Geometry check sheet. Reference: the model listing, model coordinates, mm. Round coordinates to 2 decimals unless told otherwise and drop trailing zeros. Loops run counter-clockwise (first coordinate to the right, second up) from the corner with the lowest first, then second, coordinate; pieces in that order, holes last. Notation, with made-up numbers: (85, 2) -> (141, 2) arc R10 cw to (141, 21) -> close; hole circle Ø10 at (36.5, -18.75). An arc over 180 degrees is marked (long way). Use a Markdown table: item, result. Add a question column.
Q1. Gauge pin test, flat ends, axial feed: P1, Ø2.5, axis at x = -25, z = 1.5, coming from the +Y side; P2, Ø3, axis at x = 4.5, z = 3, coming from the +Y side; P3, Ø2.5, axis at y = -17.5, z = 1.5, coming from the +X side. Record the tip position at first contact, or that the pin passes through.
Q2. Sectioned sample at D-D, the plane y = 51.5. Enter the section's corners in (x, z), then the cut area to 3 significant figures.
Q3. Material ranges on L1, parallel to Y at x = 0, z = 2.6; L2, parallel to Y at x = 11, z = 1.4; L3, parallel to X at y = 11.5, z = 2.3, recorded low to high.
Q4. Sectioned sample at A-A, the plane y = 0. Enter the section's corners in (x, z), then the cut area to 3 significant figures.
Q5. Sectioned sample at C-C, the plane z = 3.65. Enter the section's corners in (x, y), then the cut area to 3 significant figures.
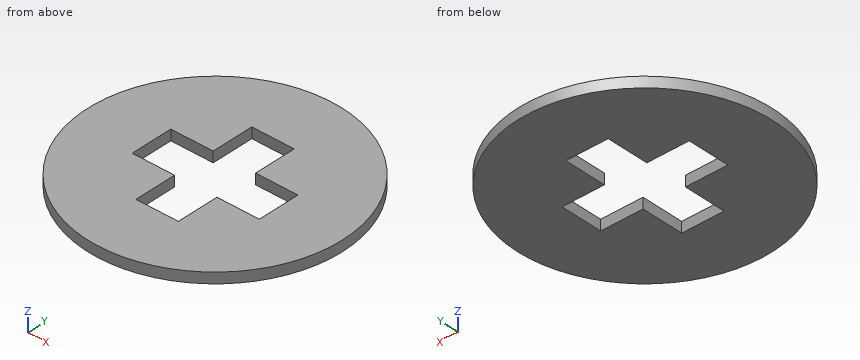
```python
from build123d import *

# Parameters (mm, degrees)
F0_R     = 60
F1_DEPTH = 5


with BuildPart() as f1:
    # F0 (on Top) → F1 (new body)
    with BuildSketch(Plane.XY):
        Circle(F0_R)
        Polygon((-10, 30), (0, 30), (10, 30), (10, 10), (30, 10), (30, 0), (30, -10), (10, -10), (10, -30), (0, -30), (-10, -30), (-10, -10), (-30, -10), (-30, 0), (-30, 10), (-10, 10), align=None, mode=Mode.SUBTRACT)
    extrude(amount=F1_DEPTH)


solid = f1.part
```
Values:
| question | item | result |
|---|---|---|
| 1 | P1 | y = 55.1 |
| 1 | P2 | y = 59.92 |
| 1 | P3 | x = 57.76 |
| 2 | outline | (-30.79, 0) -> (30.79, 0) -> (30.79, 5) -> (-30.79, 5) -> close |
| 2 | area | 308 mm^2 |
| 3 | L1 | -60 to -30, 30 to 60 |
| 3 | L2 | -58.98 to -10, 10 to 58.98 |
| 3 | L3 | -58.89 to -10, 10 to 58.89 |
| 4 | outline | (-60, 0) -> (-30, 0) -> (-30, 5) -> (-60, 5) -> close; (30, 0) -> (60, 0) -> (60, 5) -> (30, 5) -> close |
| 4 | area | 300 mm^2 |
| 5 | outline | circle Ø120 at (0, 0); hole (-30, -10) -> (-10, -10) -> (-10, -30) -> (10, -30) -> (10, -10) -> (30, -10) -> (30, 10) -> (10, 10) -> (10, 30) -> (-10, 30) -> (-10, 10) -> (-30, 10) -> close |
| 5 | area | 9,310 mm^2 |
